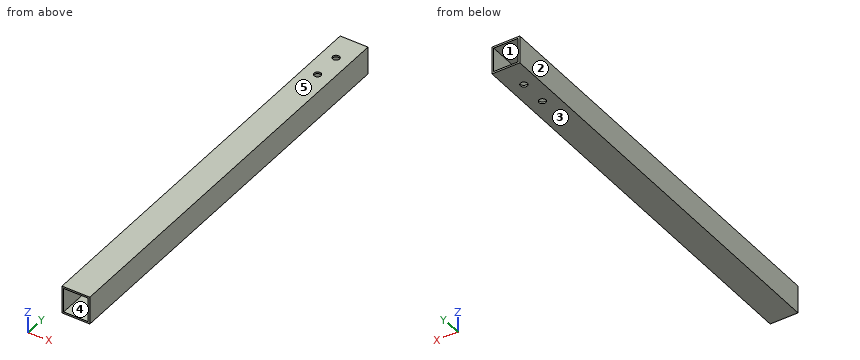
```python
from build123d import *

# Parameters (mm, degrees)
SKETCH1_W           = 25.4
SKETCH1_H           = 25.4
SKETCH1_W_2         = 22.225
SKETCH1_H_2         = 22.225
BOSS_EXTRUDE1_DEPTH = 381
SKETCH2_R           = 3.175
CUT_EXTRUDE1_DEPTH  = 26.4


with BuildPart() as part:
    # Sketch1 → Boss-Extrude1 (new body)
    with BuildSketch(Plane(origin=(0, 0, 0), x_dir=(1, 0, 0), z_dir=(0, 1, 0))):
        Rectangle(SKETCH1_W, SKETCH1_H)
        Rectangle(SKETCH1_W_2, SKETCH1_H_2, mode=Mode.SUBTRACT)
    extrude(amount=BOSS_EXTRUDE1_DEPTH)

    # Sketch2 → Cut-Extrude1 (cut, through all)
    with BuildSketch(Plane.XY.offset(12.7)):
        with Locations((0, 356.362)):
            Circle(SKETCH2_R)
        with Locations((0, 330.962)):
            Circle(SKETCH2_R)
    extrude(amount=-CUT_EXTRUDE1_DEPTH, mode=Mode.SUBTRACT)


solid = part.part
```
CAD build for the part. Positions are in the model's coordinates, mm. Face numbers are marked on the shaded views. A direction names the side the tool comes from. Coordinates: 2 decimals unless noted, no trailing zeros. Write each loop counter-clockwise with the first axis right and the second up, starting at its lowest first coordinate (ties: lowest second). Pieces come first, ordered by that corner, then holes.
(1) Cut at A-A, the plane x = 0. List the corners of the cut face in (y, z).
(2) 3-axis set-ups, long thin cutter, end or side, ignore diameter. For the marked faces 1 and 2: which of +Z, -Z, +X, -X, +Y, -Y reach the whole face in a straight line?
(3) Two-plate mould, pull along Z, no slides. Class the marked faces 3, 4 and 5: +Z half, -Z half, draft (parallel to the pull), parting line (faces both ways), or undercut.
(4) Cut at B-B, the plane y = 248.5. List the corners of the cut face in (x, z), and give its area (3 significant figures).
(5) Drill centre lines: probe 1 along Y at (x, z) = (0, -11.85); probe 2 along Z at (x, y) = (8.75, 359). Where is each one in solid material? Low to high.
(6) Cut at C-C, the plane z = -1.5. List the corners of the cut face in (x, y).
Geometry says:
1. outline: (0, -12.7) - (327.79, -12.7) - (327.79, -11.11) - (0, -11.11) - close; (0, 11.11) - (327.79, 11.11) - (327.79, 12.7) - (0, 12.7) - close; (334.14, -12.7) - (353.19, -12.7) - (353.19, -11.11) - (334.14, -11.11) - close; (334.14, 11.11) - (353.19, 11.11) - (353.19, 12.7) - (334.14, 12.7) - close; (359.54, -12.7) - (381, -12.7) - (381, -11.11) - (359.54, -11.11) - close; (359.54, 11.11) - (381, 11.11) - (381, 12.7) - (359.54, 12.7) - close
2. face 1: +Y, -Y
2. face 2: +Z, -Z, -X, +Y, -Y
3. face 3: -Z half
3. face 4: undercut
3. face 5: +Z half
4. outline: (-12.7, -12.7) - (12.7, -12.7) - (12.7, 12.7) - (-12.7, 12.7) - close; hole (-11.11, -11.11) - (11.11, -11.11) - (11.11, 11.11) - (-11.11, 11.11) - close
4. area: 151 mm2
5. probe 1: y = 0 to 327.79, 334.14 to 353.19, 359.54 to 381
5. probe 2: z = -12.7 to -11.11, 11.11 to 12.7
6. outline: (-12.7, 0) - (-11.11, 0) - (-11.11, 381) - (-12.7, 381) - close; (11.11, 0) - (12.7, 0) - (12.7, 381) - (11.11, 381) - close
